```python
from build123d import *

# Parameters (mm, degrees)
SKETCH1_R           = 28.575
SKETCH1_R_2         = 11
SKETCH1_R_3         = 3.302
BOSS_EXTRUDE1_DEPTH = 3.175
SKETCH1_4_R         = 11
BOSS_EXTRUDE2_DEPTH = 3.175
SKETCH1_5_R         = 11
BOSS_EXTRUDE3_DEPTH = 24.825
FILLET1_R           = 5


with BuildPart() as part:
    # Sketch1 → Boss-Extrude1 (new body)
    with BuildSketch(Plane(origin=(0, 0, 0), x_dir=(1, 0, 0), z_dir=(0, 1, 0))):
        Circle(SKETCH1_R)
        Circle(SKETCH1_R_2, mode=Mode.SUBTRACT)
        with Locations((21.548, 0)):
            Circle(SKETCH1_R_3, mode=Mode.SUBTRACT)
        with Locations((0, -21.548)):
            Circle(SKETCH1_R_3, mode=Mode.SUBTRACT)
        with Locations((-21.548, 0)):
            Circle(SKETCH1_R_3, mode=Mode.SUBTRACT)
        with Locations((0, 21.548)):
            Circle(SKETCH1_R_3, mode=Mode.SUBTRACT)
    extrude(amount=BOSS_EXTRUDE1_DEPTH)

    # Sketch1_4 → Boss-Extrude2 (add)
    with BuildSketch(Plane(origin=(0, 0, 0), x_dir=(1, 0, 0), z_dir=(0, 1, 0))):
        Circle(SKETCH1_4_R)
    extrude(amount=BOSS_EXTRUDE2_DEPTH)

    # Sketch1_5 → Boss-Extrude3 (add)
    with BuildSketch(Plane(origin=(0, 0, 0), x_dir=(1, 0, 0), z_dir=(0, 1, 0))):
        Circle(SKETCH1_5_R)
        with BuildLine():
            ThreePointArc((-5.414213562, -2.585786438), (-1.325654296, 5.851721173), (6, 0))
            ThreePointArc((6, 0), (3.200412581, -5.075170865), (-2.585786438, -5.414213562))
            Line((-2.585786438, -5.414213562), (-3.889087297, -6.717514421))
            Line((-3.889087297, -6.717514421), (-6.717514421, -3.889087297))
            Line((-6.717514421, -3.889087297), (-5.414213562, -2.585786438))
        make_face(mode=Mode.SUBTRACT)
    extrude(amount=-BOSS_EXTRUDE3_DEPTH)

    # Fillet1
    fillet1_edges = [part.edges().sort_by_distance(p)[0] for p in [
        (-11, 0, 0),
    ]]
    fillet(fillet1_edges, radius=FILLET1_R)


solid = part.part
```
Verification items for the finished model (mm, model axes). A direction names the side the tool comes from. Coordinates: 2 decimals unless noted, no trailing zeros. Write each loop counter-clockwise with the first axis right and the second up, starting at its lowest first coordinate (ties: lowest second). Pieces come first, ordered by that corner, then holes. Notation, with made-up numbers: (48.25, -35.5) - (69.25, -35.5) arc R26 ccw to (69.25, 1.5) - close; hole circle Ø7 at (80.5, 7.25). An arc over 180 degrees is marked (long way). One line per question, with ' | ' between items. Start each with the question number.
1. Gauge pin test, flat ends, axial feed: P1, Ø6, axis at y = -18.5, z = -15, coming from the +X side (3 decimals); P2, Ø7.5, axis at x = -21.548, z = 0, coming from the -Y side; P3, Ø12, axis at x = -22.5, y = -5.5, coming from the -Z side; P4, Ø3, axis at y = -7.5, z = 5.5, coming from the +X side. Record the tip position at first contact, or that the pin passes through.
2. Section check B-B (y = -18). Enter the section's corners in (x, z), plus the area to 3 significant figures.
3. Section check A-A (x = 0). Enter the section's corners in (y, z) (3 decimals).
4. Section check D-D (x = 23). Enter the section's corners in (y, z) (3 decimals).
5. Material ranges on line 1 along X through (y, z) = (0.9, 0) (3 decimals); line 2 along Z through (x, y) = (0, -16.5); line 3 along Y through (x, z) = (18, 22) (3 decimals), recorded low to high.
6. Access from +Z, -Z, +X, -X, +Y, -Y to the whole of each face (thin tool, end or side, straight path). Record for faces 1 (the flat face through (-6.075, -12.239, 3.247)), 2 (the cylindrical face through (-28.547, 1.565, -1.256)).
7. Section check C-C (z = 23.5). Enter the section's corners in (x, y) (3 decimals).
8. Draft check along Z on faces 3 (the cylindrical face through (-2.38, -14.77, 10.74)), 4 (the cylindrical face through (24.7, 1.57, -0.99)), 5 (the flat face through (0, 3.175, 0)). Enter one of: released by +Z, released by -Z, zero draft, split by the parting line, or undercut.
Computed values:
1) P1: through | P2: y = 0 | P3: z = -20.31 | P4: x = 10.25
2) outline: circle Ø22 at (0, 0); hole (-6.72, 3.89) - (-5.41, 2.59) arc R6 ccw (long way) to (-2.59, 5.41) - (-3.89, 6.72) - close | area: 261 mm²
3) outline: (-24.825, -11) - (-5, -11) arc R5 cw to (0, -16) - (0, -18.246) - (3.175, -18.246) - (3.175, 18.246) - (0, 18.246) - (0, 16) arc R5 cw to (-5, 11) - (-24.825, 11) - (-24.825, 6) - (0, 6) - (0, -6) - (-24.825, -6) - close; (0, -28.575) - (3.175, -28.575) - (3.175, -24.85) - (0, -24.85) - close; (0, 24.85) - (3.175, 24.85) - (3.175, 28.575) - (0, 28.575) - close
4) outline: (0, -16.957) - (3.175, -16.957) - (3.175, -2.966) - (0, -2.966) - close; (0, 2.966) - (3.175, 2.966) - (3.175, 16.957) - (0, 16.957) - close
5) line 1: -28.575 to -24.85, -18.246 to 18.246, 24.85 to 28.575 | line 2: -11 to -6, 6 to 11 | line 3: 0 to 3.175
6) face 1: -Y | face 2: +Y, -Y
7) outline: (-16.257, 0) - (-2.663, 0) - (-2.663, 3.175) - (-16.257, 3.175) - close; (2.663, 0) - (16.257, 0) - (16.257, 3.175) - (2.663, 3.175) - close
8) face 3: split by the parting line | face 4: undercut | face 5: zero draft
